from build123d import *

# Parameters (mm, degrees)
RESSALTO_EXTRUS_O1_DEPTH = 0.45
ESBO_O2_R                = 0.5
CORTE_EXTRUS_O1_DEPTH    = 16.978422951


with BuildPart() as part:
    # Esboço1 → Ressalto-extrusão1 (new, symmetric)
    with BuildSketch(Plane(origin=(0, 0, 0), x_dir=(1, 0, 0), z_dir=(0, 1, 0))):
        with BuildLine():
            Line((12.5, -8.5), (-12.5, -8.5))
            ThreePointArc((-12.5, -8.5), (-13.207106781, -8.207106781), (-13.5, -7.5))
            Line((-13.5, -7.5), (-13.5, 7.5))
            ThreePointArc((-13.5, 7.5), (-13.207106781, 8.207106781), (-12.5, 8.5))
            Line((-12.5, 8.5), (12.5, 8.5))
            ThreePointArc((12.5, 8.5), (13.207106781, 8.207106781), (13.5, 7.5))
            Line((13.5, 7.5), (13.5, -7.5))
            ThreePointArc((13.5, -7.5), (13.207106781, -8.207106781), (12.5, -8.5))
        make_face()
    extrude(amount=RESSALTO_EXTRUS_O1_DEPTH, both=True)

    # Esboço2 → Corte-extrusão1 (cut, through all)
    with BuildSketch(Plane(origin=(0, 0.45, 0), x_dir=(1, 0, 0), z_dir=(0, 1, 0))):
        with Locations(Location((-12.3, 3.8, 0), (0, 0, 270))):
            Circle(ESBO_O2_R)
        with Locations(Location((-12.3, 6.8, 0), (0, 0, 270))):
            Circle(ESBO_O2_R)
        with Locations(Location((-12.3, -6.8, 0), (0, 0, 90))):
            Circle(ESBO_O2_R)
        with Locations(Location((-12.3, -3.8, 0), (0, 0, 90))):
            Circle(ESBO_O2_R)
    extrude(amount=-CORTE_EXTRUS_O1_DEPTH, mode=Mode.SUBTRACT)


solid = part.part
The model under review builds one solid part; all positions refer to its coordinate system, in mm. Coordinates: 2 decimals unless noted, no trailing zeros. Loops run counter-clockwise (first coordinate to the right, second up) from the corner with the lowest first, then second, coordinate; pieces in that order, holes last.
(1) Draft analysis for pull direction X (two halves, no side actions). For faces 1 (the cylindrical face through (-12.3, 0, 7.3)), 2 (the flat face through (-13.5, 0, 0)), 3 (the cylindrical face through (13.199, 0.006, -8.215)), state which applies: +X half, -X half, draft (parallel to the pull), parting line (faces both ways), or undercut.
Determined:
face 1: undercut
face 2: -X half
face 3: +X half
(2) Wall thickness on L1, parallel to X at y = -0.2, z = -3.8; L2, parallel to Z at x = 12.75, y = 0.4: over which ranges is each line inside the solid? List them lowest first.
Determined:
L1: x = -13.5 to -12.8, -11.8 to 13.5
L2: z = -8.47 to 8.47
(3) Consider section B-B, the plane z = -4. Give the boundary of the cut face in (x, y).
Determined:
outline: (-13.5, -0.45) - (-12.76, -0.45) - (-12.76, 0.45) - (-13.5, 0.45) - close; (-11.84, -0.45) - (13.5, -0.45) - (13.5, 0.45) - (-11.84, 0.45) - close
(4) Consider section A-A, the plane z = 6.8. Give the boundary of the cut face in (x, y).
Determined:
outline: (-13.5, -0.45) - (-12.8, -0.45) - (-12.8, 0.45) - (-13.5, 0.45) - close; (-11.8, -0.45) - (13.5, -0.45) - (13.5, 0.45) - (-11.8, 0.45) - close
